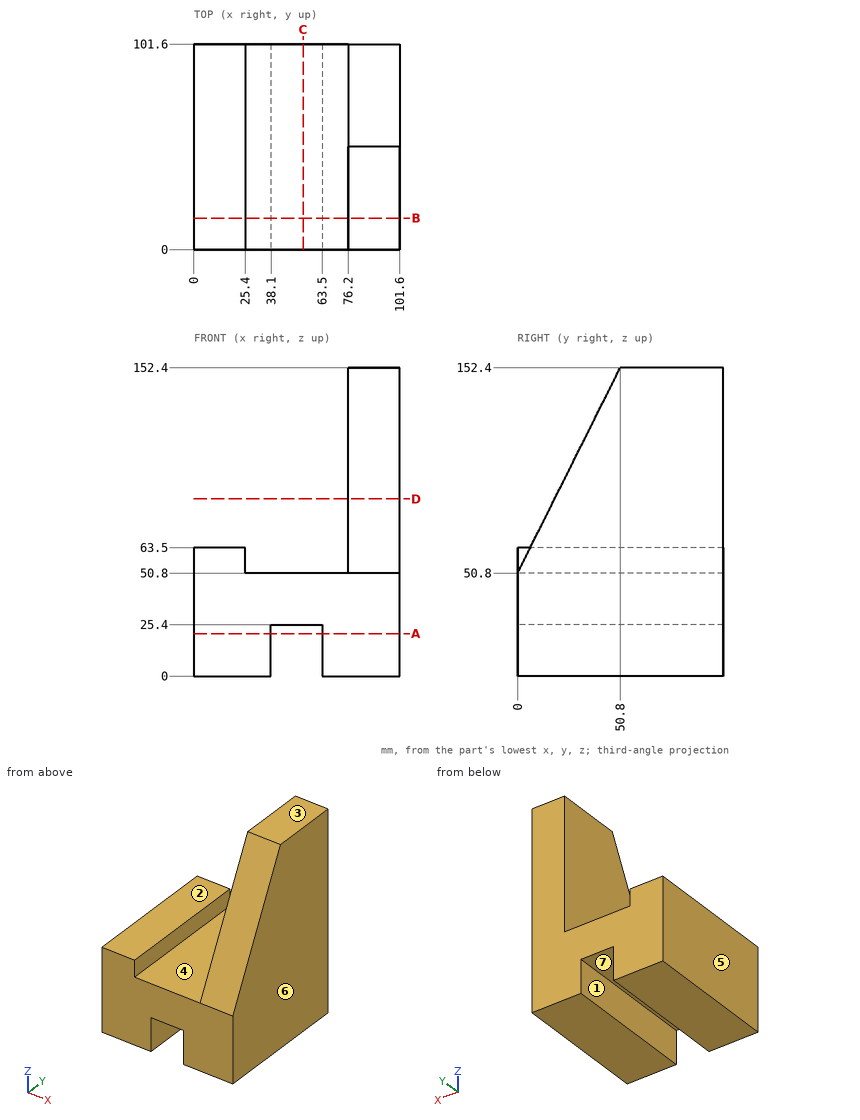
The figure shows three views and two pictorial views of one solid part (mm, origin at its lowest corner). Answer the questions. A direction names the side the tool comes from. Round coordinates to 2 decimals unless told otherwise and drop trailing zeros. Loops run counter-clockwise (first coordinate to the right, second up) from the corner with the lowest first, then second, coordinate; pieces in that order, holes last. Notation, with made-up numbers: M 64.25,85 L 80.25,85 A9 cw 80.25,96 Z; hole C -35.75,84.5 d7. An arc over 180 degrees is marked long. Write each question's results on one line, items separated by ' | '. Start each with the question number.
1) Determine the mould class of the marked faces 5, 6 and 7 for opening direction X: pulls with the +X half, pulls with the -X half, needs draft (parallel to the pull), parting line crosses it, or undercut.
2) Find section D-D on z = 87.5. Write down the section's boundary in (x, y).
3) Straight lines are drawn through the part: probe 1 along X at (y, z) = (46.5, 51); probe 2 along X at (y, z) = (87.5, 67); probe 3 along Z at (x, y) = (5, 64). For each, find the intervals that lie inside material, in ascending order.
4) Find section B-B on y = 15.5. Write down the section's boundary in (x, z).
5) Find section C-C on x = 54. Write down the section's boundary in (y, z).
6) Each of these flat-tipped pins is pushed along its axis until it touches: pin 1 (7.5 mm diameter, centred on x = 8.5, y = 35.5, fed in from +Z); pin 2 (5 mm diameter, centred on x = 44, y = 42.5, fed in from -Z). Where does it stop, or does it pass through?
7) Find section A-A on z = 21. Write down the section's boundary in (x, y), plus the area to 3 significant figures.
8) Which of the six approach directions +Z, -Z, +X, -X, +Y, -Y give full straight-line access (tool end or side, diameter ignored) to the marked faces 1, 2, 3 and 4?
Final values:
1) face 5: pulls with the -X half | face 6: pulls with the +X half | face 7: undercut
2) outline: M 76.2,18.35 L 101.6,18.35 L 101.6,101.6 L 76.2,101.6 Z
3) probe 1: 0 to 25.4, 76.2 to 101.6 | probe 2: 76.2 to 101.6 | probe 3: 0 to 63.5
4) outline: M 0,0 L 38.1,0 L 38.1,25.4 L 63.5,25.4 L 63.5,0 L 101.6,0 L 101.6,81.8 L 76.2,81.8 L 76.2,50.8 L 25.4,50.8 L 25.4,63.5 L 0,63.5 Z
5) outline: M 0,25.4 L 101.6,25.4 L 101.6,50.8 L 0,50.8 Z
6) pin 1: z = 63.5 | pin 2: z = 25.4
7) outline: M 0,0 L 38.1,0 L 38.1,101.6 L 0,101.6 Z; M 63.5,0 L 101.6,0 L 101.6,101.6 L 63.5,101.6 Z | area: 7,740 mm²
8) face 1: -Z, +Y, -Y | face 2: +Z, -X, +Y, -Y | face 3: +Z, +X, -X, +Y, -Y | face 4: +Z, +Y, -Y
